Geometry check sheet. Reference: the model listing, model coordinates, mm. Round coordinates to 2 decimals unless told otherwise and drop trailing zeros. Order: outer loops, then holes, each group sorted by start corner. A loop starts at its lowest first (then second) coordinate and runs counter-clockwise, first axis right, second up.
(1) Sectioned sample at C-C (x = 27.5). Record the boundary of the cut face in (y, z).
(2) Sectioned sample at B-B (z = 0.85). Record the boundary of the cut face in (x, y).
(3) Sectioned sample at D-D (x = 17). Record the boundary of the cut face in (y, z), plus the area to 3 significant figures.
(4) Go/stop test with a flat-tipped pin: pin 1 (11 mm diameter, centred on x = 24.97, y = -8.11, fed in from -Z). Record where the tip stops, or that it passes through.
(5) Material ranges on line 1 along Y through (x, z) = (25.5, 0.35); line 2 along X through (y, z) = (-5.75, 0.1); line 3 along Y through (x, z) = (26, 0.9), recorded low to high.
(6) Sectioned sample at A-A (y = -7.25). Record the boundary of the cut face in (x, z), plus the area to 3 significant figures.
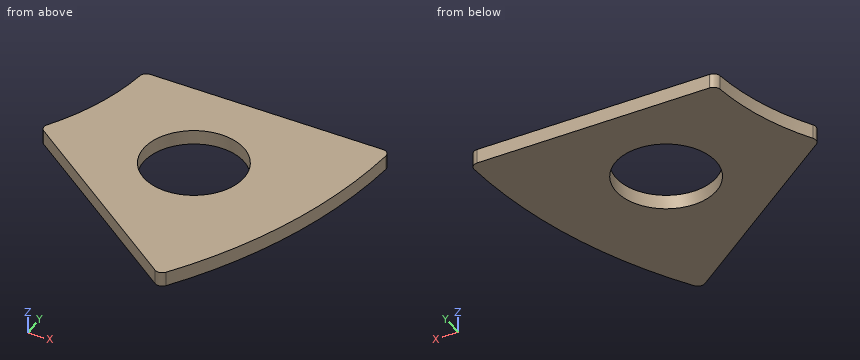
from build123d import *

# Parameters (mm, degrees)
BOSS_EXTRUDE1_DEPTH  = 1.016
M6_CLEARANCE_HOLE1_D = 7
FILLET2_R            = 0.5


with BuildPart() as part:
    # Sketch1 → Boss-Extrude1 (new body)
    with BuildSketch(Plane.XY):
        with BuildLine():
            Line((17.465394356, -1.1), (34.982710015, -1.1))
            ThreePointArc((34.982710015, -1.1), (33.28697807, -10.815594803), (28.948170689, -19.672402338))
            Line((28.948170689, -19.672402338), (14.776364625, -9.375982534))
            ThreePointArc((14.776364625, -9.375982534), (16.643489035, -5.407797402), (17.465394356, -1.1))
        make_face()
    extrude(amount=BOSS_EXTRUDE1_DEPTH)

    # M6 Clearance Hole1 (through all)
    with Locations(Plane.XY.offset(1.016)):
        with Locations((24.965233553, -8.111696102)):
            Hole(M6_CLEARANCE_HOLE1_D / 2)

    # Fillet2
    fillet2_edges = [part.edges().sort_by_distance(p)[0] for p in [
        (17.465394356, -1.1, 0.508),
        (34.982710015, -1.1, 0.508),
        (28.948170689, -19.672402338, 0.508),
        (14.776364625, -9.375982534, 0.508),
    ]]
    fillet(fillet2_edges, radius=FILLET2_R)


solid = part.part
Answer below:
1. outline: (-18.62, 0) - (-10.53, 0) - (-10.53, 1.02) - (-18.62, 1.02) - close; (-5.7, 0) - (-1.1, 0) - (-1.1, 1.02) - (-5.7, 1.02) - close
2. outline: (15.02, -8.99) arc R0.5 ccw to (15.15, -9.65) - (28.53, -19.37) arc R0.5 ccw to (29.24, -19.24) arc R35 ccw to (34.96, -1.62) arc R0.5 ccw to (34.46, -1.1) - (17.93, -1.1) arc R0.5 ccw to (17.43, -1.56) arc R17.5 cw to start; hole circle Ø7 at (24.97, -8.11)
3. outline: (-10.99, 0) - (-4.15, 0) - (-4.15, 1.02) - (-10.99, 1.02) - close
3. area: 6.95 mm2
4. pin 1: stops at z = 0
5. line 1: y = -17.17 to -11.57, -4.65 to -1.1
5. line 2: x = 16.53 to 22.38, 27.55 to 34.52
5. line 3: y = -17.53 to -11.46, -4.77 to -1.1
6. outline: (15.93, 0) - (21.57, 0) - (21.57, 1.02) - (15.93, 1.02) - close; (28.36, 0) - (34.24, 0) - (34.24, 1.02) - (28.36, 1.02) - close
6. area: 11.7 mm2
